The listing builds one solid part. Answer for the finished solid, in the listing's coordinates (mm). Face numbers are marked on the shaded views. A direction names the side the tool comes from. Coordinates: 2 decimals unless noted, no trailing zeros. Write each loop counter-clockwise with the first axis right and the second up, starting at its lowest first coordinate (ties: lowest second). Pieces come first, ordered by that corner, then holes.
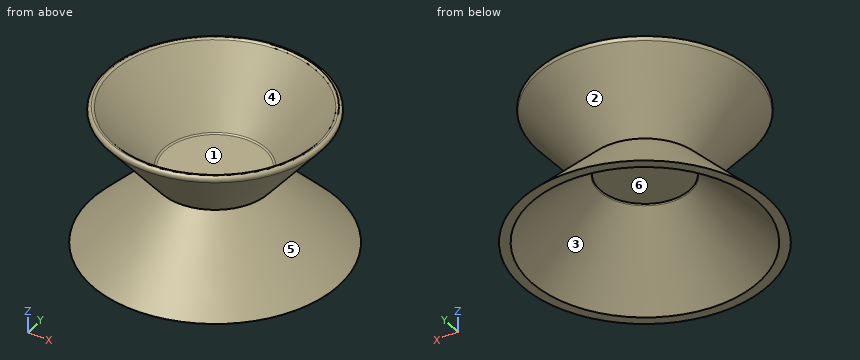
from build123d import *

# Parameters (mm, degrees)
F0_R      = 49.2737208463
F1_DEPTH  = 63.5
F1_TAPER  = -40
F2_T      = -6.35
F3_R      = 3.17499
F1_FACE_R = 49.2737208463
F4_DEPTH  = 63.5
F4_TAPER  = -45
F5_T      = -6.35
F6_R      = 2.286


# Not quite as in the source:
# - a fillet or chamfer that OpenCascade refuses, or shapes differently, is made with other operations: its cross-section is extruded or revolved along the edge and cut away or added
# - a fillet or chamfer is up to 0.001 mm smaller than in the source, because OpenCascade refuses the exact size


with BuildPart() as f1:
    # F0 (on Top) → F1 (new body)
    with BuildSketch(Plane.XY):
        Circle(F0_R)
    extrude(amount=F1_DEPTH, taper=F1_TAPER)

    # F2
    f2_openings = [f1.faces().sort_by_distance(p)[0] for p in [
        (0, 0, 63.5),
    ]]
    offset(amount=F2_T, openings=f2_openings, kind=Kind.INTERSECTION)

    # F3 (radius 3.175 in the source; OpenCascade refuses exactly that, so slightly less here)
    f3_edges = [f1.edges().sort_by_distance(p)[0] for p in [
        (-102.556547, 0, 63.5),
        (-94.267211, 0, 63.5),
    ]]
    fillet(f3_edges, radius=F3_R)

    # F1_face (on face) → F4 (join)
    with BuildSketch(Plane(origin=(0, 0, 0), x_dir=(1, 0, 0), z_dir=(0, 0, -1))):
        Circle(F1_FACE_R)
    extrude(amount=F4_DEPTH, taper=F4_TAPER)

    # F5
    f5_openings = [f1.faces().sort_by_distance(p)[0] for p in [
        (0, 0, -63.5),
    ]]
    offset(amount=F5_T, openings=f5_openings, kind=Kind.INTERSECTION)

    # F6
    f6_edges = [f1.edges().sort_by_distance(p)[0] for p in [
        (-46.312667, 0, 6.35),
    ]]
    fillet(f6_edges, radius=F6_R)

    # F7: fillet of radius 2.286 on 1 edges, made by hand

    # F7_s1 → F7_t2 (revolve, cut)
    with BuildSketch(Plane.XZ):
        with BuildLine():
            ThreePointArc((41.6376699139, -1.3442051886), (41.1980722658, -0.7269988473), (40.984384559, 0))
            Line((40.984384559, 0), (40.6691484685, -0.3756837433))
            Line((40.6691484685, -0.3756837433), (41.6376699139, -1.3442051886))
        make_face()
    revolve(axis=Axis((0, 0, -0.3756837433), (0, 0, 1)), mode=Mode.SUBTRACT)


solid = f1.part
Q1. Determine the mould class of the marked faces 4, 5 and 6 for opening direction Z: released by +Z, released by -Z, zero draft, split by the parting line, or undercut.
Answers below:
face 4: released by +Z
face 5: undercut
face 6: released by -Z
Q2. The part is cut by section B-B, the plane z = -25. Write down the section's boundary in (x, y).
Answers below:
outline: circle Ø148.55 at (0, 0); hole circle Ø130.59 at (0, 0)
Q3. Find the intervals of material crossed by probe 1 along Y at (x, z) = (-7, 15); probe 2 along Y at (x, z) = (40, 18); probe 3 along X at (y, z) = (-40.5, -6), in increasing order.
Answers below:
probe 1: y = -61.46 to -53.11, 53.11 to 61.46
probe 2: y = -50.44 to -39.32, 39.32 to 50.44
probe 3: x = -37.62 to -22.42, 22.42 to 37.62
Q4. Given pin 1 (4 mm diameter, centred on y = 14, z = -45, fed in from -X); pin 2 (12 mm diameter, centred on x = -63, y = 33.5, fed in from +Z); pin 3 (1.5 mm diameter, centred on x = 66, y = -5, fed in from +Z), each flat-ended and moving along its own axis, determine where each tip first touches the part or whether it passes through.
Answers below:
pin 1: stops at x = -95.27
pin 2: stops at z = 43.34
pin 3: stops at z = 30.93
Q5. The part is cut by section C-C, the plane z = 35. Write down the section's boundary in (x, y), then the cut area to 3 significant figures.
Answers below:
outline: circle Ø157.28 at (0, 0); hole circle Ø140.71 at (0, 0)
area: 3,880 mm2
Q6. Which of the six approach directions +Z, -Z, +X, -X, +Y, -Y give full straight-line access (tool end or side, diameter ignored) to the marked faces 1, 2 and 3?
Answers below:
face 1: +Z
face 2: none
face 3: -Z
